The figure shows three views and two pictorial views of one solid part (mm, origin at its lowest corner). Answer the questions. Coordinates: 2 decimals unless noted, no trailing zeros. Order: outer loops, then holes, each group sorted by start corner. A loop starts at its lowest first (then second) coordinate and runs counter-clockwise, first axis right, second up.
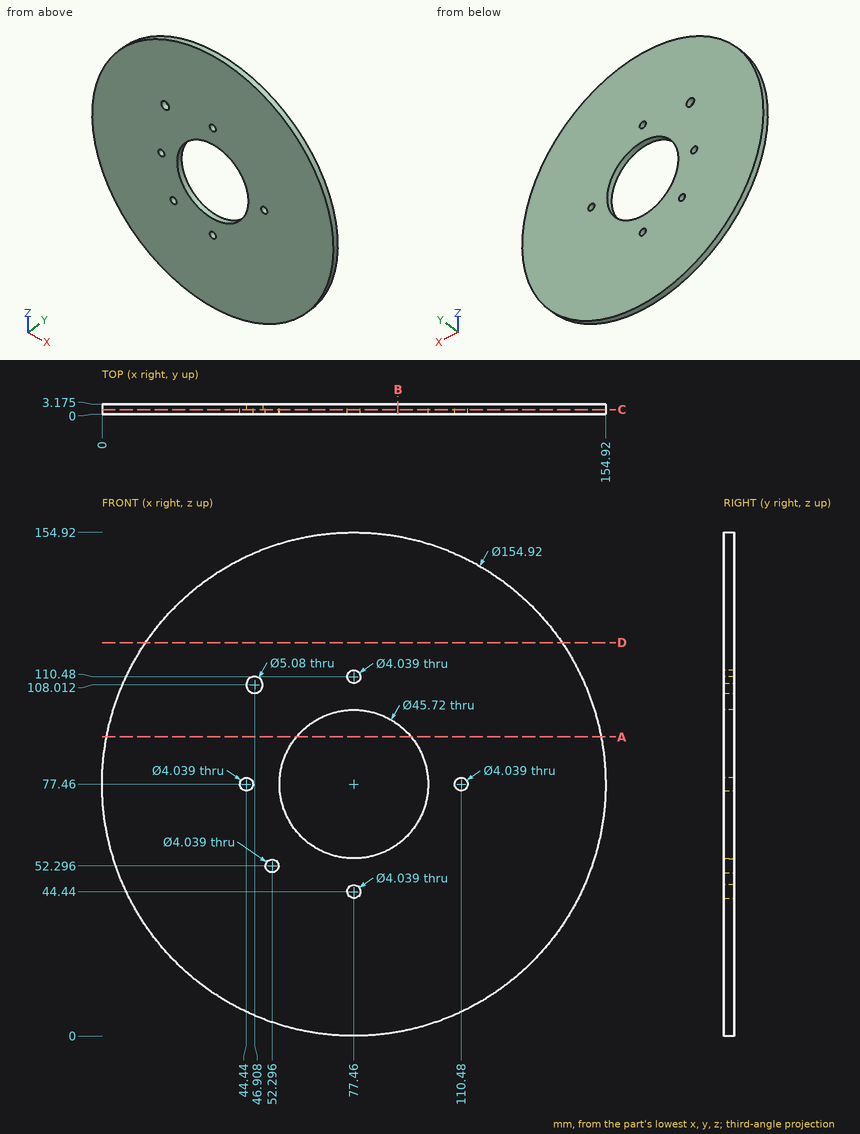
Q1. The part is cut by section A-A, the plane z = 92. Determine the outline of the cut face in (x, y) (1 decimal).
Q2. The part is cut by section D-D, the plane z = 121. Determine the outline of the cut face in (x, y) (1 decimal).
Q3. Each of these flat-tipped pins is pushed along its axis until it touches: P1, Ø1.5, axis at x = 52, z = 36, coming from the -Y side; P2, Ø1.5, axis at x = 138.5, y = 1.5, coming from the +Z side. Where does it stop, or does it pass through?
Q4. The part is cut by section C-C, the plane y = 1.45. Determine the outline of the cut face in (x, z) (1 decimal), then the cut area to 3 significant figures.
Q5. The part is cut by section B-B, the plane x = 91. Determine the outline of the cut face in (y, z) (1 decimal).
Q6. Straight lines are drawn through the part: L1, parallel to Z at x = 83, y = 1.55; L2, parallel to X at y = 0.55, z = 69; L3, parallel to Z at x = 80, y = 1.85. For each, find the intervals that lie inside material, in ascending order.
Computed values:
1. outline: (1.4, 0) - (59.8, 0) - (59.8, 3.2) - (1.4, 3.2) - close; (95.1, 0) - (153.5, 0) - (153.5, 3.2) - (95.1, 3.2) - close
2. outline: (13.4, 0) - (141.5, 0) - (141.5, 3.2) - (13.4, 3.2) - close
3. P1: stops at y = 0
3. P2: stops at z = 126.09
4. outline: circle Ø154.9 at (77.5, 77.5); hole circle Ø4 at (44.4, 77.5); hole circle Ø5.1 at (46.9, 108); hole circle Ø4 at (52.3, 52.3); hole circle Ø45.7 at (77.5, 77.5); hole circle Ø4 at (77.5, 44.4); hole circle Ø4 at (77.5, 110.5); hole circle Ø4 at (110.5, 77.5)
4. area: 17,100 mm2
5. outline: (0, 1.2) - (3.2, 1.2) - (3.2, 59) - (0, 59) - close; (0, 95.9) - (3.2, 95.9) - (3.2, 153.7) - (0, 153.7) - close
6. L1: z = 0.2 to 55.28, 99.64 to 154.72
6. L2: x = 0.46 to 56.22, 98.7 to 154.46
6. L3: z = 0.04 to 54.74, 100.18 to 154.88
